Verification items for the finished model (mm, model axes). A direction names the side the tool comes from. Round coordinates to 2 decimals unless told otherwise and drop trailing zeros. Write each loop counter-clockwise with the first axis right and the second up, starting at its lowest first coordinate (ties: lowest second). Pieces come first, ordered by that corner, then holes. Notation, with made-up numbers: (60.25, 42.5) - (106.25, 42.5) arc R35 cw to (106.25, 78.5) - close; hole circle Ø4 at (9, 23.5). An arc over 180 degrees is marked (long way). Answer as a JSON object with one key per item and string values.
```python
from build123d import *

# Parameters (mm, degrees)
F1_DEPTH       = 25
F3_D           = 6.7564
F3_CSINK_D     = 13.716
F3_CSINK_ANGLE = 82
F4_SIZE        = 1.25
F5_SIZE        = 1


with BuildPart() as f1:
    # F0 (on Top) → F1 (new body)
    with BuildSketch(Plane.XY):
        Polygon((-12.5, 10), (-12.5, 0), (12.5, 0), (12.5, 10), (7, 10), (7, 8.5), (10, 8.5), (10, 6), (-10, 6), (-10, 8.5), (-7, 8.5), (-7, 10), align=None)
    extrude(amount=F1_DEPTH)

    # F3 (through all)
    with Locations(Plane(origin=(0, 6, 0), x_dir=(-1, 0, 0), z_dir=(0, 1, 0))):
        with Locations((0, 12.5)):
            CounterSinkHole(F3_D / 2, F3_CSINK_D / 2, counter_sink_angle=F3_CSINK_ANGLE)

    # F4
    f4_edges = [f1.edges().sort_by_distance(p)[0] for p in [
        (-10, 7.25, 25),
        (10, 7.25, 25),
    ]]
    chamfer(f4_edges, length=F4_SIZE)

    # F5
    f5_edges = [f1.edges().sort_by_distance(p)[0] for p in [
        (12.5, 10, 12.5),
        (12.5, 0, 12.5),
        (-12.5, 10, 12.5),
        (-12.5, 0, 12.5),
    ]]
    chamfer(f5_edges, length=F5_SIZE)


solid = f1.part
```
1. Cross-section at C-C (y = 8). Record the boundary of the cut face in (x, z), plus the area to 3 significant figures.
Completed:
{"outline": "(-12.5, 0) - (-10, 0) - (-10, 23.75) - (-11.25, 25) - (-12.5, 25) - close; (10, 0) - (12.5, 0) - (12.5, 25) - (11.25, 25) - (10, 23.75) - close", "area": "123 mm^2"}
2. Cross-section at D-D (z = 3). Record the boundary of the cut face in (x, y).
Completed:
{"outline": "(-12.5, 1) - (-11.5, 0) - (11.5, 0) - (12.5, 1) - (12.5, 9) - (11.5, 10) - (7, 10) - (7, 8.5) - (10, 8.5) - (10, 6) - (-10, 6) - (-10, 8.5) - (-7, 8.5) - (-7, 10) - (-11.5, 10) - (-12.5, 9) - close"}
3. Go/stop test with a flat-tipped pin: pin 1 (1 mm diameter, centred on x = -1.5, y = 7, fed in from +Z). Record where the tip stops, or that it passes through.
Completed:
{"pin 1": "passes through"}
4. Mould release check, pull along Z, two halves, no side actions. Record for faces 5 (the face through (1.91, 2.19, 15.49)), 6 (the face through (10.62, 7.27, 24.37)), 7 (the face through (7, 9, 12)): released by +Z, released by -Z, zero draft, split by the parting line, or undercut.
Completed:
{"face 5": "undercut", "face 6": "released by +Z", "face 7": "zero draft"}
5. Access from +Z, -Z, +X, -X, +Y, -Y to the whole of each face (thin tool, end or side, straight path). Record for faces 1 (the face through (-7, 9, 12)), 2 (the face through (-10.62, 7.23, 24.37)), 3 (the face through (-10, 7, 12)), 4 (the face through (9, 10, 12)).
Completed:
{"face 1": "+Z, -Z, +Y", "face 2": "+Z", "face 3": "+Z, -Z", "face 4": "+Z, -Z, +X, -X, +Y"}
6. Cross-section at B-B (z = 12.5). Record the boundary of the cut face in (x, y).
Completed:
{"outline": "(-12.5, 1) - (-11.5, 0) - (-3.38, 0) - (-3.38, 2) - (-6.86, 6) - (-10, 6) - (-10, 8.5) - (-7, 8.5) - (-7, 10) - (-11.5, 10) - (-12.5, 9) - close; (3.38, 0) - (11.5, 0) - (12.5, 1) - (12.5, 9) - (11.5, 10) - (7, 10) - (7, 8.5) - (10, 8.5) - (10, 6) - (6.86, 6) - (3.38, 2) - close"}
7. Cross-section at A-A (x = -8.75). Record the boundary of the cut face in (y, z).
Completed:
{"outline": "(0, 0) - (6, 0) - (6, 25) - (0, 25) - close; (8.5, 0) - (10, 0) - (10, 25) - (8.5, 25) - close"}
8. Material ranges on probe 1 along Y at (x, z) = (-9, 23.5); probe 2 along Z at (x, y) = (0, 0.5); probe 3 along X at (y, z) = (8.25, 9), recorded low to high. Write a range as from..to.
Completed:
{"probe 1": "y = 0..6, 8.5..10", "probe 2": "z = 0..9.12, 15.88..25", "probe 3": "x = -12.5..-10, 10..12.5"}
